Check sheet for the modelled part. Datum: model origin and axes. Units: mm. Face numbers are marked on the shaded views. A direction names the side the tool comes from. Give positions to 0.01 mm unless a question says otherwise; leave off trailing zeros. Order: outer loops, then holes, each group sorted by start corner. A loop starts at its lowest first (then second) coordinate and runs counter-clockwise, first axis right, second up.
```python
from build123d import *

# Parameters (mm, degrees)
SKETCH1_W           = 9
SKETCH1_H           = 27.215298634
BOSS_EXTRUDE1_DEPTH = 4
SKETCH2_W           = 2.5
SKETCH2_H           = 27.215298634
BOSS_EXTRUDE2_DEPTH = 43.5
FILLET1_R           = 1.25
CUT_EXTRUDE1_REACH  = 57.921
SKETCH7_R           = 1.4
CUT_EXTRUDE2_DEPTH  = 75.363842374


with BuildPart() as part:
    # Sketch1 → Boss-Extrude1 (new body)
    with BuildSketch(Plane.XY):
        with Locations((-48.865, -14.497649317)):
            Rectangle(SKETCH1_W, SKETCH1_H)
    extrude(amount=BOSS_EXTRUDE1_DEPTH)

    # Sketch2 → Boss-Extrude2 (add)
    with BuildSketch(Plane.XY.offset(4)):
        with Locations((-52.115, -14.497649317)):
            Rectangle(SKETCH2_W, SKETCH2_H)
    extrude(amount=BOSS_EXTRUDE2_DEPTH)

    # Fillet1
    fillet1_edges = [part.edges().sort_by_distance(p)[0] for p in [
        (-50.865, -14.497649317, 4),
        (-53.365, -14.497649317, 47.5),
        (-44.365, -14.497649317, 4),
        (-53.365, -14.497649317, 0),
    ]]
    fillet(fillet1_edges, radius=FILLET1_R)

    # Sketch6 → Cut-Extrude1 (cut, up to next)
    with BuildSketch(Plane.ZY.offset(53.365), mode=Mode.PRIVATE) as cut_extrude1_sk1:
        with BuildLine():
            Line((6.25, -20.35), (41.25, -20.35))
            ThreePointArc((41.25, -20.35), (42.9, -22), (41.25, -23.65))
            Line((41.25, -23.65), (6.25, -23.65))
            ThreePointArc((6.25, -23.65), (4.6, -22), (6.25, -20.35))
        make_face()
    cut_extrude1_tool1 = extrude(cut_extrude1_sk1.sketch, amount=-CUT_EXTRUDE1_REACH, mode=Mode.PRIVATE) & part.part
    # Sketch6 → Cut-Extrude1 (cut, up to next)
    with BuildSketch(Plane.ZY.offset(53.365), mode=Mode.PRIVATE) as cut_extrude1_sk2:
        with BuildLine():
            Line((6.25, -5.35), (41.25, -5.35))
            ThreePointArc((41.25, -5.35), (42.9, -7), (41.25, -8.65))
            Line((41.25, -8.65), (6.25, -8.65))
            ThreePointArc((6.25, -8.65), (4.6, -7), (6.25, -5.35))
        make_face()
    cut_extrude1_tool2 = extrude(cut_extrude1_sk2.sketch, amount=-CUT_EXTRUDE1_REACH, mode=Mode.PRIVATE) & part.part
    add(cut_extrude1_tool1.solids().sort_by_distance((-53.365, -22, 23.75))[0], mode=Mode.SUBTRACT)
    add(cut_extrude1_tool2.solids().sort_by_distance((-53.365, -7, 23.75))[0], mode=Mode.SUBTRACT)

    # Sketch7 → Cut-Extrude2 (cut, through all)
    with BuildSketch(Plane.XY.offset(4)):
        with Locations((-47.5, -23.25)):
            Circle(SKETCH7_R)
        with Locations((-47.5, -5.65)):
            Circle(SKETCH7_R)
    extrude(amount=-CUT_EXTRUDE2_DEPTH, mode=Mode.SUBTRACT)


solid = part.part
```
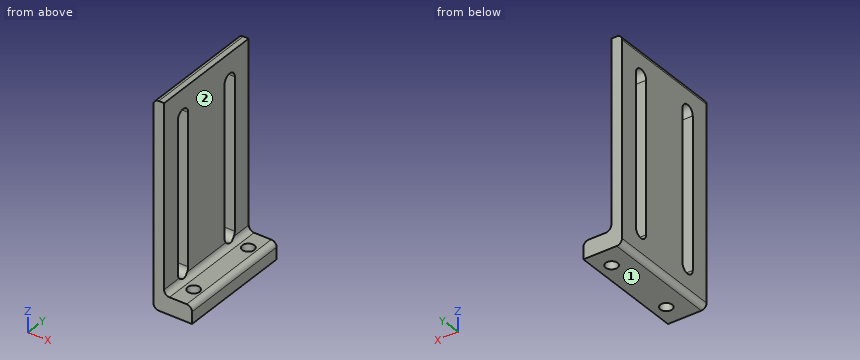
(1) Cross-section at A-A on z = 39. Enter the section's corners in (x, y) (3 decimals), then the cut area to 3 significant figures.
Response values:
outline: (-53.365, -28.105) - (-50.865, -28.105) - (-50.865, -23.65) - (-53.365, -23.65) - close; (-53.365, -20.35) - (-50.865, -20.35) - (-50.865, -8.65) - (-53.365, -8.65) - close; (-53.365, -5.35) - (-50.865, -5.35) - (-50.865, -0.89) - (-53.365, -0.89) - close
area: 51.5 mm2
(2) Set-up check for the marked faces 1 and 2: record each of +Z, -Z, +X, -X, +Y, -Y from which the full face is reachable in a straight line by a thin tool's end or side.
Response values:
face 1: -Z, +X, -X, +Y, -Y
face 2: +Z, +X, +Y, -Y
(3) Cross-section at D-D on y = -22.5. Enter the section's corners in (x, z) (3 decimals).
Response values:
outline: (-53.365, 1.25) arc R1.25 ccw to (-52.115, 0) - (-48.682, 0) - (-48.682, 4) - (-49.615, 4) arc R1.25 cw to (-50.726, 4.678) - (-53.365, 4.678) - close; (-53.365, 42.822) - (-50.865, 42.822) - (-50.865, 47.5) - (-52.115, 47.5) arc R1.25 ccw to (-53.365, 46.25) - close; (-46.318, 0) - (-44.365, 0) - (-44.365, 2.75) arc R1.25 ccw to (-45.615, 4) - (-46.318, 4) - close
(4) Material ranges on L1, parallel to Y at x = -47.5, z = 3.2; L2, parallel to Y at x = -52.5, z = 36.5; L3, parallel to X at y = -17.5, z = 43 (3 decimals), recorded low to high.
Response values:
L1: y = -28.11 to -24.65, -21.85 to -7.05, -4.25 to -0.89
L2: y = -28.11 to -23.65, -20.35 to -8.65, -5.35 to -0.89
L3: x = -53.365 to -50.865
(5) Gauge pin test, flat ends, axial feed: pin 1 Ø4 at (x, y) = (-48, -11.5) entering from +Z; pin 2 Ø3 at (y, z) = (-16, 11.5) entering from +X (3 decimals); pin 3 Ø1.7 at (x, y) = (-47.5, -5.65) entering from -Z; pin 4 Ø2 at (x, y) = (-47.5, -18.5) entering from +Z. Record the tip position at first contact, or that the pin passes through.
Response values:
pin 1: stops at z = 4.06
pin 2: stops at x = -50.865
pin 3: passes through
pin 4: stops at z = 4
(6) Cross-section at C-C on y = -19. Enter the section's corners in (x, z) (3 decimals), then the cut area to 3 significant figures.
Response values:
outline: (-53.365, 1.25) arc R1.25 ccw to (-52.115, 0) - (-44.365, 0) - (-44.365, 2.75) arc R1.25 ccw to (-45.615, 4) - (-49.615, 4) arc R1.25 cw to (-50.865, 5.25) - (-50.865, 47.5) - (-52.115, 47.5) arc R1.25 ccw to (-53.365, 46.25) - close
area: 144 mm2
(7) Cross-section at B-B on x = -47.5. Enter the section's corners in (y, z), then the cut area to 3 significant figures.
Response values:
outline: (-28.11, 0) - (-24.65, 0) - (-24.65, 4) - (-28.11, 4) - close; (-21.85, 0) - (-7.05, 0) - (-7.05, 4) - (-21.85, 4) - close; (-4.25, 0) - (-0.89, 0) - (-0.89, 4) - (-4.25, 4) - close
area: 86.5 mm2
